Input: part model. Units: mm. Frame: model coordinates. A direction names the side the tool comes from. Coordinates: 2 decimals unless noted, no trailing zeros. Write each loop counter-clockwise with the first axis right and the second up, starting at its lowest first coordinate (ties: lowest second). Pieces come first, ordered by that corner, then holes.
1) Section query A-A (z = -12). Output: boundary loops of the cut face in (x, y), then the cut area to 3 significant figures.
2) Set-up query: faces 1 (the cylindrical face through (26.56, 98.83, 1.27)), 2 (the flat face through (19, 53, -2)), 3 (the flat face through (18, 49.595, -1)), 4 (the cylindrical face through (-0.545, 51.272, 0.646)), 5 (the cylindrical face through (36.997, 79.459, -1.141)). Return all of +Z, -Z, +X, -X, +Y, -Y with unobstructed straight access to the full face (end or side cutting, diameter ignored); none if empty.
3) Section query C-C (x = 28.5). Output: boundary loops of the cut face in (y, z).
4) Section query B-B (y = 100.41). Output: boundary loops of the cut face in (x, z) (3 decimals), then the cut area to 3 significant figures.
5) Draft query along Y for faces 6 (the flat face through (0, 51, -19)), 7 (the cylindrical face through (26.028, 3.924, 1.268)), 8 (the cylindrical face through (6.978, 3.924, 1.268)), 9 (the flat face through (22.4, 0, 0.4)). Return one class per face: pulls with the +Y half, pulls with the -Y half, needs draft (parallel to the pull), parting line crosses it, or undercut.
6) Section query D-D (y = 70). Output: boundary loops of the cut face in (x, z), then the cut area to 3 significant figures.
7) Pin query (flat end, axial travel): pin 1 Ø4 at (x, y) = (9.575, 100.41) entering from -Z; pin 2 Ø1 at (x, y) = (26, 83) entering from -Z; pin 3 Ø12 at (x, y) = (30.5, 72.5) entering from -Z; pin 4 Ø6.5 at (x, y) = (16, 53.5) entering from -Z. Return the tip coordinate at first contact, or that it passes through.
8) Line query: L1, parallel to X at y = 6, z = -25.5; L2, parallel to X at y = 3, z = 1; L3, parallel to X at y = 100, z = 1. Output: solid intervals per line, ascending.
from build123d import *

# Parameters (mm, degrees)
BOSS_EXTRUDE1_DEPTH = 104
SKETCH2_R           = 2.6
CUT_EXTRUDE1_DEPTH  = 108
SKETCH3_W           = 30.2
SKETCH3_H           = 6
BOSS_EXTRUDE2_DEPTH = 2
CHAMFER1_SIZE       = 2
FILLET1_R           = 3


with BuildPart() as part:
    # Sketch1 → Boss-Extrude1 (new body)
    with BuildSketch(Plane(origin=(0, 0, 0), x_dir=(1, 0, 0), z_dir=(0, 1, 0))):
        with BuildLine():
            Line((4, 0), (34.2, 0))
            ThreePointArc((34.2, 0), (37.028427125, 1.171572875), (38.2, 4))
            Line((38.2, 4), (38.2, 34))
            Line((38.2, 34), (40.7, 34))
            Line((40.7, 34), (40.7, 4))
            ThreePointArc((40.7, 4), (38.796194078, -0.596194078), (34.2, -2.5))
            Line((34.2, -2.5), (4, -2.5))
            ThreePointArc((4, -2.5), (-0.596194078, -0.596194078), (-2.5, 4))
            Line((-2.5, 4), (-2.5, 34))
            Line((-2.5, 34), (0, 34))
            Line((0, 34), (0, 4))
            ThreePointArc((0, 4), (1.171572875, 1.171572875), (4, 0))
        make_face()
    extrude(amount=BOSS_EXTRUDE1_DEPTH)

    # Sketch2 → Cut-Extrude1 (cut)
    with BuildSketch(Plane.XY.offset(2.5)):
        with Locations((9.575, 3.81)):
            Circle(SKETCH2_R)
        with Locations((28.625, 3.81)):
            Circle(SKETCH2_R)
        with Locations((9.575, 100.41)):
            Circle(SKETCH2_R)
        with Locations((28.625, 100.41)):
            Circle(SKETCH2_R)
    extrude(amount=-CUT_EXTRUDE1_DEPTH, mode=Mode.SUBTRACT)

    # Sketch3 → Boss-Extrude2 (add)
    with BuildSketch(Plane(origin=(0, 0, 0), x_dir=(-1, 0, 0), z_dir=(0, 0, -1))):
        with Locations((-19.1, 52.595312466)):
            Rectangle(SKETCH3_W, SKETCH3_H)
    extrude(amount=BOSS_EXTRUDE2_DEPTH)

    # Chamfer1
    # the kernel refuses this chamfer: 10, 2 mm, written as the material it adds along each edge
    with BuildSketch(Plane(origin=(34.2, 55.595312466, 0), x_dir=(0.908761807760111, 0, -0.41731520072551287), z_dir=(0, -1, 0))) as chamfer1_piece_1_section:
        with BuildLine():
            Line((3.338521606, 0), (CHAMFER1_SIZE * 0.417315200726, -CHAMFER1_SIZE * 0.90876180776))
            Line((CHAMFER1_SIZE * 0.417315200726, -CHAMFER1_SIZE * 0.90876180776), (0, 0))
            ThreePointArc((0, 0), (1.841628656, 0.361237209), (3.338521606, 0))
        make_face()
    chamfer1_piece_1 = extrude(amount=6, mode=Mode.PRIVATE)
    chamfer1_piece_1 = split(chamfer1_piece_1, bisect_by=Plane(origin=(34.2, 55.595312466, -2), z_dir=(0, 0, 1)), keep=Keep.TOP, mode=Mode.PRIVATE)
    add(chamfer1_piece_1)
    with BuildSketch(Plane(origin=(4, 49.595312466, 0), x_dir=(-0.9087618077601108, 0, -0.41731520072551315), z_dir=(0, 1, 0))) as chamfer1_piece_2_section:
        with BuildLine():
            Line((3.338521606, 0), (CHAMFER1_SIZE * 0.417315200726, -CHAMFER1_SIZE * 0.90876180776))
            Line((CHAMFER1_SIZE * 0.417315200726, -CHAMFER1_SIZE * 0.90876180776), (0, 0))
            ThreePointArc((0, 0), (1.841628656, 0.361237209), (3.338521606, 0))
        make_face()
    chamfer1_piece_2 = extrude(amount=6, mode=Mode.PRIVATE)
    chamfer1_piece_2 = split(chamfer1_piece_2, bisect_by=Plane(origin=(4, 49.595312466, -2), z_dir=(0, 0, 1)), keep=Keep.TOP, mode=Mode.PRIVATE)
    add(chamfer1_piece_2)

    # Fillet1
    # the kernel refuses this fillet: 3 mm, written as the material it adds along each edge
    with BuildSketch(Plane(origin=(37.23392093, 55.595312466, -1.393215814), x_dir=(-0.9805806756909838, 0, -0.1961161351378653), z_dir=(0, -1, 0)), Plane(origin=(0.96607907, 49.595312466, -1.393215814), x_dir=(0.9805806756909838, 0, -0.19611613513786538), z_dir=(0, 1, 0))) as fillet1_piece_1:
        with BuildLine():
            CenterArc((2.674200502, 3), FILLET1_R, 168.690067526, 101.309932474)
            Line((-0.267541525, 3.588348405), (-0.561715728, 3.647183246))
            ThreePointArc((-0.561715728, 3.647183246), (-0.730260231, 2.804460732), (-0.261467751, -0.147087101))
            Line((-0.261467751, -0.147087101), (0, -0.3))
            Line((0, -0.3), (2.674200502, -0.3))
            Line((2.674200502, -0.3), (2.674200502, 0))
        make_face()
    extrude(amount=6)


solid = part.part
Answer:
1. outline: (-2.5, 0) - (0, 0) - (0, 104) - (-2.5, 104) - close; (38.2, 0) - (40.7, 0) - (40.7, 104) - (38.2, 104) - close
1. area: 520 mm2
2. face 1: +Z, -Z
2. face 2: -Z, +Y, -Y
2. face 3: -Z, -Y
2. face 4: +Z, -X, +Y, -Y
2. face 5: -Z, +Y
3. outline: (0, 0) - (1.21, 0) - (1.21, 2.5) - (0, 2.5) - close; (6.41, 0) - (49.6, 0) - (49.6, -2) - (55.6, -2) - (55.6, 0) - (97.81, 0) - (97.81, 2.5) - (6.41, 2.5) - close; (103.01, 0) - (104, 0) - (104, 2.5) - (103.01, 2.5) - close
4. outline: (-2.5, -34) - (0, -34) - (0, -4) arc R4 cw to (4, 0) - (6.975, 0) - (6.975, 2.5) - (4, 2.5) arc R6.5 ccw to (-2.5, -4) - close; (12.175, 0) - (26.025, 0) - (26.025, 2.5) - (12.175, 2.5) - close; (31.225, 0) - (34.2, 0) arc R4 cw to (38.2, -4) - (38.2, -34) - (40.7, -34) - (40.7, -4) arc R6.5 ccw to (34.2, 2.5) - (31.225, 2.5) - close
4. area: 241 mm2
5. face 6: needs draft
5. face 7: undercut
5. face 8: undercut
5. face 9: pulls with the -Y half
6. outline: (-2.5, -34) - (0, -34) - (0, -4) arc R4 cw to (4, 0) - (34.2, 0) arc R4 cw to (38.2, -4) - (38.2, -34) - (40.7, -34) - (40.7, -4) arc R6.5 ccw to (34.2, 2.5) - (4, 2.5) arc R6.5 ccw to (-2.5, -4) - close
6. area: 267 mm2
7. pin 1: passes through
7. pin 2: stops at z = 0
7. pin 3: stops at z = -0.73
7. pin 4: stops at z = -2
8. L1: x = -2.5 to 0, 38.2 to 40.7
8. L2: x = -0.15 to 7.1, 12.05 to 26.15, 31.1 to 38.35
8. L3: x = -0.15 to 7.01, 12.14 to 26.06, 31.19 to 38.35
